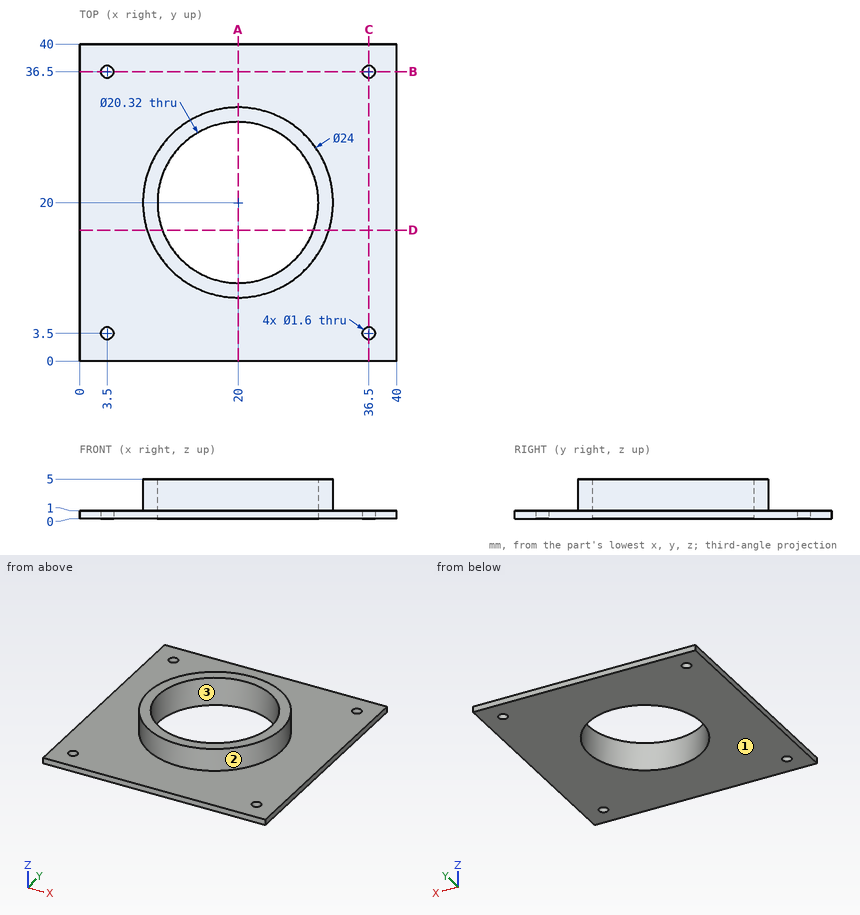
Answer from the drawing. Dimensions are ordinates in mm from the lowest x, y and z of the part. Give positions to 0.01 mm unless a question says otherwise; leave off trailing zeros. Loops run counter-clockwise (first coordinate to the right, second up) from the corner with the lowest first, then second, coordinate; pieces in that order, holes last. Notation, with made-up numbers: M 27.5,54.5 L 38.5,54.5 A24 cw 38.5,73.5 Z; hole C 47.5,77.25 d2. An arc over 180 degrees is marked long. One line per item, written item: value.
Q1. A cutting plane is placed at D-D on y = 16.5. Determine the outline of the cut face in (x, z), then the cut area to 3 significant figures.
Working result:
outline: M 0,0 L 10.46,0 L 10.46,5 L 8.52,5 L 8.52,1 L 0,1 Z; M 29.54,0 L 40,0 L 40,1 L 31.48,1 L 31.48,5 L 29.54,5 Z
area: 36.4 mm^2
Q2. A cutting plane is placed at A-A on x = 20. Determine the outline of the cut face in (y, z), then the cut area to 3 significant figures.
Working result:
outline: M 0,0 L 9.84,0 L 9.84,5 L 8,5 L 8,1 L 0,1 Z; M 30.16,0 L 40,0 L 40,1 L 32,1 L 32,5 L 30.16,5 Z
area: 34.4 mm^2
Q3. Flat-ended cylindrical pins translate along their axes: P1, Ø1.5, axis at y = 19.5, z = 2.5, coming from the +X side; P2, Ø3, axis at x = 19, z = 3, coming from the -Y side; P3, Ø1.8, axis at x = 3.5, y = 3.5, coming from the +Z side; P4, Ø16.5, axis at x = 20, y = 20, coming from the +Z side. Find the tip coordinate at first contact, or state that the pin passes through.
Working result:
P1: stops at x = 32
P2: stops at y = 8
P3: stops at z = 1
P4: passes through
Q4. Determine the mould class of the marked faces 1, 2 and 3 for opening direction X: +X half, -X half, draft (parallel to the pull), parting line (faces both ways), or undercut.
Working result:
face 1: draft
face 2: parting line
face 3: undercut
Q5. Find the intervals of material crossed by line 1 (X direction, y = 36.5, z = 0.65); line 2 (Y direction, x = 20, z = 2.7), in increasing order. Write a range as from..to.
Working result:
line 1: x = 0..2.7, 4.3..35.7, 37.3..40
line 2: y = 8..9.84, 30.16..32
Q6. A cutting plane is placed at B-B on y = 36.5. Determine the outline of the cut face in (x, z), then the cut area to 3 significant figures.
Working result:
outline: M 0,0 L 2.7,0 L 2.7,1 L 0,1 Z; M 4.3,0 L 35.7,0 L 35.7,1 L 4.3,1 Z; M 37.3,0 L 40,0 L 40,1 L 37.3,1 Z
area: 36.8 mm^2
